CAD build for the part. Positions are in the model's coordinates, mm. Face numbers are marked on the shaded views. A direction names the side the tool comes from. Round coordinates to 2 decimals unless told otherwise and drop trailing zeros. Write each loop counter-clockwise with the first axis right and the second up, starting at its lowest first coordinate (ties: lowest second). Pieces come first, ordered by that corner, then holes. Notation, with made-up numbers: (-15.5, 79.25) -> (18.5, 79.25) arc R15 cw to (18.5, 84.25) -> close; hole circle Ø5 at (70, 68.25). An arc over 180 degrees is marked (long way). Put each result on its own line as item: value. Start each with the question number.
1. Saw through at A-A on z = 13.5. List the corners of the cut face in (x, y).
2. Saw through at D-D on z = 3.5. List the corners of the cut face in (x, y), and give its area (3 significant figures).
3. Flat gauge pins, fed straight in: P1, Ø2.5, axis at x = -12.5, y = -12.5, coming from the -Z side; P2, Ø5, axis at x = -12.5, y = 12.5, coming from the +Z side; P3, Ø2.5, axis at x = 0, y = 0, coming from the -Z side. Where does each tip first touch, or does it go through?
4. 3-axis set-ups, long thin cutter, end or side, ignore diameter. For the marked faces 1, 2 and 3: which of +Z, -Z, +X, -X, +Y, -Y reach the whole face in a straight line?
5. Drill centre lines: line 1 (Y direction, x = -31.1, z = 16); line 2 (X direction, y = 1, z = 3.75); line 3 (Y direction, x = 5, z = 17). Where is each one in solid material? Low to high. Write a range as from..to.
6. Saw through at B-B on y = -9.5. List the corners of the cut face in (x, z), and give its area (3 significant figures).
7. Pull direction X, two halves, no side cores. Call the marked faces 4, 5 and 6: pulls with the +X half, pulls with the -X half, needs draft (parallel to the pull), parting line crosses it, or undercut.
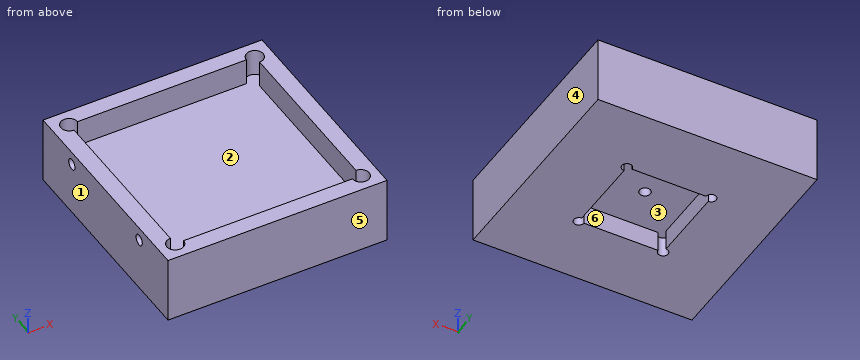
Autodesk Inventor part; units mm, degrees
ref_plane "YZ Plane" through (0, 0, 0) normal (1, 0, 0) x (0, 1, 0)
ref_plane "XZ Plane" through (0, 0, 0) normal (0, 1, 0) x (-1, 0, 0)
ref_plane "XY Plane" through (0, 0, 0) normal (0, 0, 1) x (1, 0, 0)
sketch "Sketch1" plane through (0, 0, 0) normal (0, 0, 1) x (1, 0, 0)
  line L0 (0, 45.5) -> (0, -45.5) construction
  line L1 (-45.5, 0) -> (45.5, 0) construction
  line L2 (-32.5, 32.5) -> (32.5, 32.5)
  line L3 (32.5, 32.5) -> (32.5, -32.5)
  line L4 (32.5, -32.5) -> (-32.5, -32.5)
  line L5 (-32.5, -32.5) -> (-32.5, 32.5)
  point P0 (0, 0)
  dimension "d0" = 65
  dimension "d1" = 65
extrude "Extrusion1" add sketch "Sketch1" along normal blind 20
sketch "Sketch4" plane through (0, 0, 20) normal (0, 0, 1) x (1, 0, 0)
  line L0 (-45.5, 0) -> (45.5, 0) construction
  line L1 (0, 45.5) -> (0, -45.5) construction
  line L2 (-27.55, 27.55) -> (27.55, 27.55) construction
  line L3 (27.55, 27.55) -> (27.55, -27.55) construction
  line L4 (27.55, -27.55) -> (-27.55, -27.55) construction
  line L5 (-27.55, -27.55) -> (-27.55, 27.55) construction
  point P0 (0, 0)
  dimension "d15" = 55.1
  dimension "d16" = 55.1
hole "Hole2" at (-27.55, 27.55, 20) at (27.55, 27.55, 20) at (27.55, -27.55, 20) at (-27.55, -27.55, 20) at (-27.55, 27.55, 20) at (27.55, 27.55, 20) direction (0, 0, -1) diameter 5 depth 8
sketch "Sketch5" plane through (0, 0, 20) normal (0, 0, 1) x (1, 0, 0)
  circle A0 centre (-27.55, 27.55) radius 2.5
  circle A1 centre (27.55, -27.55) radius 2.5
  line L0 (-27.55, 27.55) -> (27.55, 27.55)
  line L1 (27.55, 27.55) -> (27.55, -27.55)
  line L2 (27.55, -27.55) -> (-27.55, -27.55)
  line L3 (-27.55, -27.55) -> (-27.55, 27.55)
  point P0 (0, 0)
extrude "Extrusion3" cut sketch "Sketch5" against normal blind 8 contours L0 L1 A1 L2 L3 A0 | A0 L3 L0 | L1 L2 A1 picked at (-25.9042, 27.3646) picked at (27.003, -25.9868)
sketch "Sketch6" plane through (-32.5, -32.5, 0) normal (-1, 0, 0) x (0, 0, 1)
  line L0 (0, 65) -> (20, 65)
  line L1 (0, 0) -> (20, 0)
  line L2 (20, 7.45) -> (12, 7.45) construction
  line L3 (20, 57.55) -> (20, 7.45) construction
  line L4 (12, 57.55) -> (20, 57.55) construction
  line L5 (12, 7.45) -> (12, 57.55) construction
  line L6 (16, 57.55) -> (16, 7.45) construction
  point P0 (0, 32.5)
  point P1 (16, 50)
  point P2 (16, 15)
  dimension "d26" = 15
  dimension "d27" = 15
hole "Hole3" at (-32.5, 17.5, 16) at (-32.5, -17.5, 16) direction (1, 0, 0) diameter 3.242 end up to surface
sketch "Sketch8" plane through (0, 0, 0) normal (0, 0, -1) x (-1, 0, 0)
  line L0 (32.5, 32.5) -> (-32.5, 32.5) construction
  line L1 (-32.5, 32.5) -> (-32.5, -32.5) construction
  line L2 (-32.5, -32.5) -> (32.5, -32.5) construction
  line L3 (32.5, -32.5) -> (32.5, 32.5) construction
  line L4 (0, -45.5) -> (0, 45.5) construction
  line L5 (-45.5, 0) -> (45.5, 0) construction
  line L6 (12.5, -12.5) -> (-12.5, -12.5)
  line L7 (-12.5, -12.5) -> (-12.5, 12.5)
  line L8 (-12.5, 12.5) -> (12.5, 12.5)
  line L9 (12.5, 12.5) -> (12.5, -12.5)
  point P0 (0, 0)
  dimension "d44" = 25
  dimension "d45" = 25
extrude "Extrusion4" cut sketch "Sketch8" against normal blind 6
sketch "Sketch9" plane through (0, 0, 0) normal (0, 0, -1) x (-1, 0, 0)
  line L0 (12.5, 12.5) -> (12.5, -12.5) construction
  line L1 (12.5, -12.5) -> (-12.5, -12.5) construction
  line L2 (-12.5, -12.5) -> (-12.5, 12.5) construction
  line L3 (-12.5, 12.5) -> (12.5, 12.5) construction
  line L4 (32.5, 32.5) -> (-32.5, 32.5) construction
  line L5 (-32.5, 32.5) -> (-32.5, -32.5) construction
  line L6 (-32.5, -32.5) -> (32.5, -32.5) construction
  line L7 (32.5, -32.5) -> (32.5, 32.5) construction
  line L8 (12.5, -12.5) -> (-12.5, -12.5) construction
  point P0 (0, 0)
hole "Hole5" at (-12.5, -12.5, 0) at (12.5, -12.5, 0) at (12.5, 12.5, 0) at (-12.5, 12.5, 0) direction (0, 0, 1) diameter 3 depth 6
sketch "Sketch10" plane through (0, 0, 6) normal (0, 0, -1) x (-1, 0, 0)
  point P0 (0, 0)
  point P1 (0, 0)
hole "Hole6" at (0, 0, 6) direction (0, 0, 1) diameter 3.242 depth 4 tip angle 118
properties part number "Large-cuvette-mount-50mm-V3" material "PC/ABS Plastic"
Return value:
1. outline: (-32.5, -32.5) -> (32.5, -32.5) -> (32.5, 32.5) -> (-32.5, 32.5) -> close; hole (-27.55, -25.05) arc R2.5 ccw (long way) to (-25.05, -27.55) -> (25.05, -27.55) arc R2.5 ccw (long way) to (27.55, -25.05) -> (27.55, 25.05) arc R2.5 ccw (long way) to (25.05, 27.55) -> (-25.05, 27.55) arc R2.5 ccw (long way) to (-27.55, 25.05) -> close
2. outline: (-32.5, -32.5) -> (32.5, -32.5) -> (32.5, 32.5) -> (-32.5, 32.5) -> close; hole (-12.5, -11) arc R1.5 ccw (long way) to (-11, -12.5) -> (11, -12.5) arc R1.5 ccw (long way) to (12.5, -11) -> (12.5, 11) arc R1.5 ccw (long way) to (11, 12.5) -> (-11, 12.5) arc R1.5 ccw (long way) to (-12.5, 11) -> close
2. area: 3,580 mm^2
3. P1: stops at z = 6
3. P2: stops at z = 12
3. P3: stops at z = 10.22
4. face 1: +Z, -Z, -X, +Y, -Y
4. face 2: +Z
4. face 3: -Z
5. line 1: y = -32.5..-19.12, -15.88..15.88, 19.12..32.5
5. line 2: x = -32.5..-12.5, 12.5..32.5
5. line 3: y = -32.5..-27.55, 27.55..32.5
6. outline: (-32.5, 0) -> (-12.5, 0) -> (-12.5, 6) -> (12.5, 6) -> (12.5, 0) -> (32.5, 0) -> (32.5, 20) -> (27.55, 20) -> (27.55, 12) -> (-27.55, 12) -> (-27.55, 20) -> (-32.5, 20) -> close
6. area: 709 mm^2
7. face 4: pulls with the +X half
7. face 5: needs draft
7. face 6: undercut
